CAD build for the part. Positions are in the model's coordinates, mm. Give positions to 0.01 mm unless a question says otherwise; leave off trailing zeros. Order: outer loops, then holes, each group sorted by start corner. A loop starts at its lowest first (then second) coordinate and runs counter-clockwise, first axis right, second up.
from build123d import *

# Parameters (mm, degrees)
F0_R     = 1042.9875
F0_R_2   = 6.35
F0_R_3   = 305.59375
F0_R_4   = 85.725
F1_DEPTH = 3.048


with BuildPart() as f1:
    # F0 (on Top) → F1 (new body)
    with BuildSketch(Plane.XY):
        Circle(F0_R)
        with Locations((-534.176408, -871.696672)):
            Circle(F0_R_2, mode=Mode.SUBTRACT)
        with Locations((-871.696672, -534.176408)):
            Circle(F0_R_2, mode=Mode.SUBTRACT)
        with Locations((-663.963212, -777.401039)):
            Circle(F0_R_2, mode=Mode.SUBTRACT)
        with Locations((-777.401039, -663.963212)):
            Circle(F0_R_2, mode=Mode.SUBTRACT)
        with Locations((-391.236407, -944.52824)):
            Circle(F0_R_2, mode=Mode.SUBTRACT)
        with Locations((-238.662868, -994.102388)):
            Circle(F0_R_2, mode=Mode.SUBTRACT)
        with Locations((-80.212657, -1019.198436)):
            Circle(F0_R_2, mode=Mode.SUBTRACT)
        with Locations((-944.52824, -391.236407)):
            Circle(F0_R_2, mode=Mode.SUBTRACT)
        with Locations((-994.102388, -238.662868)):
            Circle(F0_R_2, mode=Mode.SUBTRACT)
        with Locations((-1019.198436, -80.212657)):
            Circle(F0_R_2, mode=Mode.SUBTRACT)
        with Locations((80.212657, -1019.198436)):
            Circle(F0_R_2, mode=Mode.SUBTRACT)
        with Locations((238.662868, -994.102388)):
            Circle(F0_R_2, mode=Mode.SUBTRACT)
        with Locations((391.236407, -944.52824)):
            Circle(F0_R_2, mode=Mode.SUBTRACT)
        with Locations((534.176408, -871.696672)):
            Circle(F0_R_2, mode=Mode.SUBTRACT)
        with Locations((663.963212, -777.401039)):
            Circle(F0_R_2, mode=Mode.SUBTRACT)
        with Locations((777.401039, -663.963212)):
            Circle(F0_R_2, mode=Mode.SUBTRACT)
        with Locations((871.696672, -534.176408)):
            Circle(F0_R_2, mode=Mode.SUBTRACT)
        with Locations((944.52824, -391.236407)):
            Circle(F0_R_2, mode=Mode.SUBTRACT)
        with Locations((994.102388, -238.662868)):
            Circle(F0_R_2, mode=Mode.SUBTRACT)
        with Locations((1019.198436, -80.212657)):
            Circle(F0_R_2, mode=Mode.SUBTRACT)
        with Locations((-1019.198436, 80.212657)):
            Circle(F0_R_2, mode=Mode.SUBTRACT)
        with Locations((-994.102388, 238.662868)):
            Circle(F0_R_2, mode=Mode.SUBTRACT)
        with Locations((-944.52824, 391.236407)):
            Circle(F0_R_2, mode=Mode.SUBTRACT)
        with Locations((-871.696672, 534.176408)):
            Circle(F0_R_2, mode=Mode.SUBTRACT)
        with Locations((-777.401039, 663.963212)):
            Circle(F0_R_2, mode=Mode.SUBTRACT)
        with Locations((-663.963212, 777.401039)):
            Circle(F0_R_2, mode=Mode.SUBTRACT)
        with Locations((-534.176408, 871.696672)):
            Circle(F0_R_2, mode=Mode.SUBTRACT)
        with Locations((-391.236407, 944.52824)):
            Circle(F0_R_2, mode=Mode.SUBTRACT)
        with Locations((-238.662868, 994.102388)):
            Circle(F0_R_2, mode=Mode.SUBTRACT)
        with Locations((-80.212657, 1019.198436)):
            Circle(F0_R_2, mode=Mode.SUBTRACT)
        Circle(F0_R_3, mode=Mode.SUBTRACT)
        with Locations((1019.198436, 80.212657)):
            Circle(F0_R_2, mode=Mode.SUBTRACT)
        with Locations((994.102388, 238.662868)):
            Circle(F0_R_2, mode=Mode.SUBTRACT)
        with Locations((944.52824, 391.236407)):
            Circle(F0_R_2, mode=Mode.SUBTRACT)
        with Locations((0, 873.125)):
            Circle(F0_R_4, mode=Mode.SUBTRACT)
        with Locations((80.212657, 1019.198436)):
            Circle(F0_R_2, mode=Mode.SUBTRACT)
        with Locations((238.662868, 994.102388)):
            Circle(F0_R_2, mode=Mode.SUBTRACT)
        with Locations((391.236407, 944.52824)):
            Circle(F0_R_2, mode=Mode.SUBTRACT)
        with Locations((777.401039, 663.963212)):
            Circle(F0_R_2, mode=Mode.SUBTRACT)
        with Locations((663.963212, 777.401039)):
            Circle(F0_R_2, mode=Mode.SUBTRACT)
        with Locations((871.696672, 534.176408)):
            Circle(F0_R_2, mode=Mode.SUBTRACT)
        with Locations((534.176408, 871.696672)):
            Circle(F0_R_2, mode=Mode.SUBTRACT)
    extrude(amount=F1_DEPTH)


solid = f1.part
1. Saw through at B-B on x = 0. Give the cut face in (y, z), plus the area to 3 significant figures.
2. Mould opens along Y. For faces 1 (the cylindrical face through (994.824, 313.285, 1.503)), 2 (the flat face through (217, -217, 0)), 3 (the cylindrical face through (-66.247, -298.327, 1.503)) say: released by +Y, released by -Y, zero draft, split by the parting line, or undercut.
3. Saw through at C-C on z = 0.5. State how many separate pieces and enclosed holes the cut face has, plus the area to 3 significant figures.
4. Saw through at A-A on y = 0. Give the cut face in (x, z), plus the area to 3 significant figures.
5. Wall check: line 1 (X direction, y = 127.5, z = 2.7); line 2 (Y direction, x = -392.5, z = 1.15); line 3 (X direction, y = -50, z = 0.7). Give the ranges that are in metal, low to high.
6. Pin check, flat tips, straight feed: P1, Ø14.5, axis at x = 777.4, y = 663.96, coming from the -Z side; P2, Ø1.5, axis at y = -545, z = 2.5, coming from the +X side; P3, Ø1, axis at x = 175.5, z = 2, coming from the +Y side. Stop position of each tip, or through.
7. Saw through at D-D on y = -909. Give the cut face in (x, z).
Reported:
1. outline: (-1042.99, 0) - (-305.59, 0) - (-305.59, 3.05) - (-1042.99, 3.05) - close; (305.59, 0) - (787.4, 0) - (787.4, 3.05) - (305.59, 3.05) - close; (958.85, 0) - (1042.99, 0) - (1042.99, 3.05) - (958.85, 3.05) - close
1. area: 3,970 mm2
2. face 1: split by the parting line
2. face 2: zero draft
2. face 3: undercut
3. separate pieces: 1
3. enclosed holes: 42
3. area: 3,100,000 mm2
4. outline: (-1042.99, 0) - (-305.59, 0) - (-305.59, 3.05) - (-1042.99, 3.05) - close; (305.59, 0) - (1042.99, 0) - (1042.99, 3.05) - (305.59, 3.05) - close
4. area: 4,500 mm2
5. line 1: x = -1035.17 to -277.73, 277.73 to 1035.17
5. line 2: y = -966.32 to -950.75, -938.31 to 938.31, 950.75 to 966.32
5. line 3: x = -1041.79 to -301.48, 301.48 to 1041.79
6. P1: stops at z = 0
6. P2: stops at x = 889.73
6. P3: stops at y = 1028.2
7. outline: (-511.41, 0) - (511.41, 0) - (511.41, 3.05) - (-511.41, 3.05) - close
